from build123d import *

# Parameters (mm, degrees)
SKETCH003_R  = 2.5
PAD_DEPTH    = 10
SKETCH002_W  = 35
SKETCH002_H  = 35
SKETCH002_R  = 1.5
PAD001_DEPTH = 33
SKETCH004_R  = 11
PAD002_DEPTH = 1.5
PAD003_DEPTH = 22
CHAMFER_SIZE = 2


with BuildPart() as part:
    # Sketch003 → Pad (new body)
    with BuildSketch(Plane.XY):
        Circle(SKETCH003_R)
    extrude(amount=-PAD_DEPTH)

    # Sketch002 → Pad001 (new body)
    with BuildSketch(Plane.XY):
        Rectangle(SKETCH002_W, SKETCH002_H)
        with Locations((-13, 13)):
            Circle(SKETCH002_R, mode=Mode.SUBTRACT)
        with Locations((13, 13)):
            Circle(SKETCH002_R, mode=Mode.SUBTRACT)
        with Locations((13, -13)):
            Circle(SKETCH002_R, mode=Mode.SUBTRACT)
        with Locations((-13, -13)):
            Circle(SKETCH002_R, mode=Mode.SUBTRACT)
    extrude(amount=PAD001_DEPTH)

    # Sketch004 → Pad002 (new body)
    with BuildSketch(Plane.XY.offset(33)):
        Circle(SKETCH004_R)
    extrude(amount=PAD002_DEPTH)

    # Sketch005 → Pad003 (new body)
    with BuildSketch(Plane.XY.offset(34.5)):
        with BuildLine():
            ThreePointArc((1.5, -2), (0, 2.5), (-1.5, -2))
            Line((1.5, -2), (-1.5, -2))
        make_face()
    extrude(amount=PAD003_DEPTH)

    # Chamfer
    chamfer_edges = [part.edges().sort_by_distance(p)[0] for p in [
        (-17.5, -17.5, 16.5),
        (-17.5, 17.5, 16.5),
        (17.5, -17.5, 16.5),
        (17.5, 17.5, 16.5),
    ]]
    chamfer(chamfer_edges, length=CHAMFER_SIZE)


solid = part.part
Can you work these out from the model? Positions are in its coordinate system, mm. A direction names the side the tool comes from. Coordinates: 2 decimals unless noted, no trailing zeros. Order: outer loops, then holes, each group sorted by start corner. A loop starts at its lowest first (then second) coordinate and runs counter-clockwise, first axis right, second up. Notation, with made-up numbers: (37.5, -22) - (78.5, -22) arc R23 cw to (78.5, 1) - close; hole circle Ø1 at (57, -33.5). An arc over 180 degrees is marked (long way). Answer as a JSON object with one key per item and string values. Group by question number.
Q1. Imagine slicing it at A-A (y = -13). Please give me the cut outline in (x, z).
Q2. Imagine slicing it at D-D (x = 0). Please give me the cut outline in (y, z).
Q3. On a 3-axis mill with a long thin cutter (end or side, diameter ignored), from which of +Z, -Z, +X, -X, +Y, -Y can I reach the whole of each face in a straight line? I mean faces 1 (the face through (0, -2, 45)), 2 (the face through (17, 16, 16)), 3 (the face through (-2.38, -10.74, 33.74)), 4 (the face through (-0.54, -2.44, -4.93)). Say none if no direction works.
Q4. Imagine slicing it at B-B (z = 19). Please give me the cut outline in (x, y).
Q5. Will these pins go through, and if not, where does the flat tip stop? P1, Ø17.5, axis at x = 2.5, y = -4.5, coming from the -Z side; P2, Ø12, axis at x = 6.5, y = -13.5, coming from the +Z side; P3, Ø3.5, axis at x = 13, y = 13, coming from the -Z side; P4, Ø1.8, axis at x = 13, y = -13, coming from the +Z side.
Q6. We'd pull the mould along X, two halves only. Please class faces 5 (the face through (-14.5, -12.93, 16.27)), 6 (the face through (-16, -17, 16)), 7 (the face through (-0.2, -2.3, 34.5)), 8 (the face through (11.5, 13.07, 16.27)): +X half, -X half, draft (parallel to the pull), parting line (faces both ways), or undercut.
Q7. I need wall thicknesses on line 1 (Y direction, x = 13, z = 20.5); line 2 (Z direction, x = 3, y = -15); line 3 (Z direction, x = -2, y = 7.5). Which ranges of each line are inside material? Lowest first, please. Write a range as from..to.
Determined:
{
 "1": {"outline": "(-17.5, 0) - (-14.5, 0) - (-14.5, 33) - (-17.5, 33) - close; (-11.5, 0) - (11.5, 0) - (11.5, 33) - (-11.5, 33) - close; (14.5, 0) - (17.5, 0) - (17.5, 33) - (14.5, 33) - close"},
 "2": {"outline": "(-17.5, 0) - (-2.5, 0) - (-2.5, -10) - (2.5, -10) - (2.5, 0) - (17.5, 0) - (17.5, 33) - (11, 33) - (11, 34.5) - (2.5, 34.5) - (2.5, 56.5) - (-2, 56.5) - (-2, 34.5) - (-11, 34.5) - (-11, 33) - (-17.5, 33) - close"},
 "3": {"face 1": "+Z, +X, -X, -Y", "face 2": "+Z, -Z, +X, +Y", "face 3": "+Z", "face 4": "-Z"},
 "4": {"outline": "(-17.5, -15.5) - (-15.5, -17.5) - (15.5, -17.5) - (17.5, -15.5) - (17.5, 15.5) - (15.5, 17.5) - (-15.5, 17.5) - (-17.5, 15.5) - close; hole circle Ø3 at (-13, -13); hole circle Ø3 at (-13, 13); hole circle Ø3 at (13, -13); hole circle Ø3 at (13, 13)"},
 "5": {"P1": "stops at z = -10", "P2": "stops at z = 34.5", "P3": "stops at z = 0", "P4": "passes through"},
 "6": {"face 5": "undercut", "face 6": "-X half", "face 7": "draft", "face 8": "undercut"},
 "7": {"line 1": "y = -17.5..-14.5, -11.5..11.5, 14.5..17.5", "line 2": "z = 0..33", "line 3": "z = 0..34.5"}
}
